CAD build for the part. Positions are in the model's coordinates, mm. Coordinates: 2 decimals unless noted, no trailing zeros. Order: outer loops, then holes, each group sorted by start corner. A loop starts at its lowest first (then second) coordinate and runs counter-clockwise, first axis right, second up. Notation, with made-up numbers: M 36,24.25 L 90,24.25 A23 cw 90,61.25 Z; hole C 70,11 d3. An arc over 180 degrees is marked long. One line per item, written item: value.
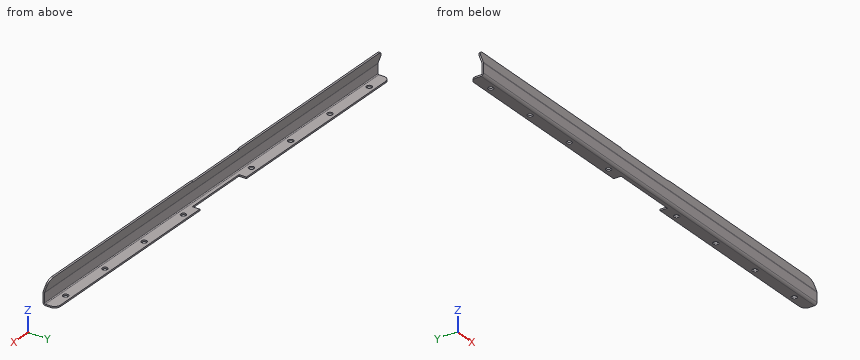
from build123d import *

# Parameters (mm, degrees)
SKETCH1_W                    = 1.25
SKETCH1_H                    = 10
BASE_FLANGE1_DEPTH           = 401
EDGE_FLANGE1_STRIP_W         = 6.4732
EDGE_FLANGE1_STRIP_H         = 1.25
EDGE_FLANGE1_STRIP_CUT_DEPTH = 401
EDGE_FLANGE1_DEPTH           = 401
EDGE_FLANGE2_STRIP_CUT_DEPTH = 401
EDGE_FLANGE2_DEPTH           = 401
CUT_EXTRUDE1_START           = 172.5
CUT_EXTRUDE1_OUTLINE_W       = 6.25
CUT_EXTRUDE1_OUTLINE_H       = 1.25
CUT_EXTRUDE1_DEPTH           = 56
SKETCH10_R                   = 2.25
CUT_EXTRUDE2_DEPTH           = 10
FILLET1_R                    = 5


# Read off the part's stored shape, not the designer's step: Cut-Extrude1
# Sheet-metal steps are written as plain solids
with BuildPart() as part:
    # Sketch1 → Base-Flange1 (new body)
    with BuildSketch(Plane(origin=(0, 0, 0), x_dir=(0, 0, -1), z_dir=(1, 0, 0))):
        with Locations((-0.625, 5)):
            Rectangle(SKETCH1_W, SKETCH1_H)
    extrude(amount=BASE_FLANGE1_DEPTH)

    # Edge-Flange1 strip (across the edge) → Edge-Flange1 strip cut (cut)
    with BuildSketch(Plane(origin=(0, 0, 1.25), x_dir=(0, 1, 0), z_dir=(1, 0, 0))):
        with Locations((-2.5, -0.625)):
            Rectangle(EDGE_FLANGE1_STRIP_W, EDGE_FLANGE1_STRIP_H)
    extrude(amount=EDGE_FLANGE1_STRIP_CUT_DEPTH, mode=Mode.SUBTRACT)

    # Edge-Flange1 section (across the edge) → Edge-Flange1 (add)
    with BuildSketch(Plane(origin=(0, 0, 1.25), x_dir=(0, 1, 0), z_dir=(1, 0, 0))):
        with BuildLine():
            Line((-1.25, 0.7366), (-1.25, 8.75))
            Line((-1.25, 8.75), (0, 8.75))
            Line((0, 8.75), (0, 0.7366))
            ThreePointArc((0, 0.7366), (0.215745145, 0.215745145), (0.7366, 0))
            Line((0.7366, 0), (0.7366, -1.25))
            ThreePointArc((0.7366, -1.25), (-0.668138332, -0.668138332), (-1.25, 0.7366))
        make_face()
    extrude(amount=EDGE_FLANGE1_DEPTH)

    # Edge-Flange2 strip (across the edge) → Edge-Flange2 strip cut (cut)
    with BuildSketch(Plane(origin=(0, 0, 10), x_dir=(0, 0.9396926207859113, -0.3420201433256607), z_dir=(1, 0, 0))):
        Polygon((-3.344158152, 5.53324351), (-1.13019336, -0.549574763), (0.044422416, -0.122049584), (-2.169542376, 5.960768689), align=None)
    extrude(amount=EDGE_FLANGE2_STRIP_CUT_DEPTH, mode=Mode.SUBTRACT)

    # Edge-Flange2 section (across the edge) → Edge-Flange2 (add)
    with BuildSketch(Plane(origin=(0, 0, 10), x_dir=(0, 0.9396926207859113, -0.3420201433256607), z_dir=(1, 0, 0))):
        with BuildLine():
            Line((-1.25, 0.129882454), (-1.25, 11.779591274))
            Line((-1.25, 11.779591274), (0, 11.779591274))
            Line((0, 11.779591274), (0, 0.129882454))
            ThreePointArc((0, 0.129882454), (0.011190609, 0.001973206), (0.044422416, -0.122049584))
            Line((0.044422416, -0.122049584), (-1.13019336, -0.549574763))
            ThreePointArc((-1.13019336, -0.549574763), (-1.219819082, -0.215087016), (-1.25, 0.129882454))
        make_face()
    extrude(amount=EDGE_FLANGE2_DEPTH)

    # Cut-Extrude1 outline → Cut-Extrude1 (cut)
    with BuildSketch(Plane.YZ.offset(CUT_EXTRUDE1_START)):
        Polygon((2.85424172, 21.496720175), (2.575384224, 20.730565502), (3.75, 20.303040323), (4.028857496, 21.069194996), align=None)
        with Locations((6.875, 0.625)):
            Rectangle(CUT_EXTRUDE1_OUTLINE_W, CUT_EXTRUDE1_OUTLINE_H)
    extrude(amount=CUT_EXTRUDE1_DEPTH, mode=Mode.SUBTRACT)

    # Sketch10 → Cut-Extrude2 (cut)
    with BuildSketch(Plane(origin=(0, 0, 0), x_dir=(-1, 0, 0), z_dir=(0, 0, -1))):
        with Locations(Location((-18, 5.25, 0), (0, 0, 90))):
            Circle(SKETCH10_R)
        with Locations(Location((-65.2, 5.25, 0), (0, 0, 90))):
            Circle(SKETCH10_R)
        with Locations(Location((-112.4, 5.25, 0), (0, 0, 90))):
            Circle(SKETCH10_R)
        with Locations(Location((-159.6, 5.25, 0), (0, 0, 90))):
            Circle(SKETCH10_R)
        with Locations(Location((-241.4, 5.25, 0), (0, 0, 90))):
            Circle(SKETCH10_R)
        with Locations(Location((-288.6, 5.25, 0), (0, 0, 90))):
            Circle(SKETCH10_R)
        with Locations(Location((-335.8, 5.25, 0), (0, 0, 90))):
            Circle(SKETCH10_R)
        with Locations(Location((-383, 5.25, 0), (0, 0, 90))):
            Circle(SKETCH10_R)
    extrude(amount=-CUT_EXTRUDE2_DEPTH, mode=Mode.SUBTRACT)

    # Fillet1
    fillet1_edges = [part.edges().sort_by_distance(p)[0] for p in [
        (401, 10, 0.625),
        (0, 10, 0.625),
        (0, 3.441549608, 21.282957586),
        (401, 3.441549608, 21.282957586),
    ]]
    fillet(fillet1_edges, radius=FILLET1_R)


solid = part.part
Q1. Pin check, flat tips, straight feed: pin 1 Ø4 at (x, y) = (245.5, 7.5) entering from +Z; pin 2 Ø10 at (x, z) = (347.5, 17) entering from +Y; pin 3 Ø2 at (x, z) = (153.5, 14) entering from -Y; pin 4 Ø3 at (x, z) = (268.5, 10.5) entering from -Y. Stop position of each tip, or through.
Recorded:
pin 1: stops at z = 1.25
pin 2: stops at y = 4.03
pin 3: stops at y = -0.24
pin 4: stops at y = -1.25
Q2. Slice it at A-A (x = 123.5). List the corners of the cut face in (y, z).
Recorded:
outline: M -1.25,1.99 A1.99 ccw 0.74,0 L 10,0 L 10,1.25 L 0.74,1.25 A0.74 cw 0,1.99 L 0,9.87 A0.74 cw 0.04,10.12 L 4.03,21.07 L 2.85,21.5 L -1.13,10.55 A1.99 ccw -1.25,9.87 Z
Q3. Drill centre lines: line 1 along Z through (x, y) = (381, 8.25); line 2 along Y through (x, z) = (93.5, 7.5); line 3 along Y through (x, z) = (383, 0.7). Where is each one in solid material? Low to high.
Recorded:
line 1: z = 0 to 1.25
line 2: y = -1.25 to 0
line 3: y = -0.78 to 3, 7.5 to 10
